Build history of the part. All positions in model axes, mm. Face numbers are marked on the shaded views. A direction names the side the tool comes from. Give positions to 0.01 mm unless a question says otherwise; leave off trailing zeros. Order: outer loops, then holes, each group sorted by start corner. A loop starts at its lowest first (then second) coordinate and runs counter-clockwise, first axis right, second up. Notation, with made-up numbers: (78, 67) - (111, 67) arc R23 ccw to (111, 100) - close; hole circle Ø3 at (88, -15.75). An arc over 180 degrees is marked (long way). Answer in a Markdown table with one row per item.
```python
from build123d import *

# Parameters (mm, degrees)
SKETCH1_W               = 50.8
SKETCH1_H               = 22.225
BOSS_EXTRUDE1_DEPTH     = 34.29
SKETCH2_R               = 18.034
CUT_EXTRUDE1_DEPTH      = 45.095938092
SKETCH3_W               = 20.32
SKETCH3_H               = 19.685
CUT_EXTRUDE2_DEPTH      = 63.289098213
SKETCH4_W               = 12.7
SKETCH4_H               = 19.05
CUT_EXTRUDE3_DEPTH      = 45.095938092
SKETCH7_W               = 68.58
SKETCH7_H               = 12.7
CUT_EXTRUDE5_DEPTH      = 49.113560718
CUT_EXTRUDE6_DEPTH      = 45.095938092
CUT_EXTRUDE6_DEPTH_BACK = 45.095938092
SKETCH9_W               = 5.08
SKETCH9_H               = 5.08
SKETCH6_W               = 33.625329213
SKETCH6_H               = 19.685
CUT_EXTRUDE4_DEPTH      = 45.095938092


with BuildPart() as part:
    # Sketch1 → Boss-Extrude1 (new, symmetric)
    with BuildSketch(Plane(origin=(0, 0, 0), x_dir=(0, 0, -1), z_dir=(1, 0, 0))):
        Rectangle(SKETCH1_W, SKETCH1_H)
    extrude(amount=BOSS_EXTRUDE1_DEPTH, both=True)

    # Sketch2 → Cut-Extrude1 (cut, through all)
    with BuildSketch(Plane(origin=(0, 0, 0), x_dir=(1, 0, 0), z_dir=(0, 0.819152044288991, 0.5735764363510473))):
        with Locations(Location((0, 0, 0), (0, 0, 233.158672775))):
            Circle(SKETCH2_R)
    extrude(amount=CUT_EXTRUDE1_DEPTH, mode=Mode.SUBTRACT)

    # Sketch3 → Cut-Extrude2 (cut, through all)
    with BuildSketch(Plane.XY.offset(25.4)):
        with Locations((0, 1.27)):
            Rectangle(SKETCH3_W, SKETCH3_H)
    extrude(amount=-CUT_EXTRUDE2_DEPTH, mode=Mode.SUBTRACT)

    # Sketch4 → Cut-Extrude3 (cut, through all)
    with BuildSketch(Plane(origin=(0, 0, 0), x_dir=(1, 0, 0), z_dir=(0, 1, 0))):
        Rectangle(SKETCH4_W, SKETCH4_H)
    extrude(amount=-CUT_EXTRUDE3_DEPTH, mode=Mode.SUBTRACT)

    # Sketch7 → Cut-Extrude5 (cut, through all)
    with BuildSketch(Plane(origin=(0, 11.1125, 0), x_dir=(1, 0, 0), z_dir=(0, 1, 0))):
        with Locations((0, 19.05)):
            Rectangle(SKETCH7_W, SKETCH7_H)
    extrude(amount=-CUT_EXTRUDE5_DEPTH, mode=Mode.SUBTRACT)

    # Sketch9 → Cut-Extrude6 (cut, two sides: drawn at the far end of the back side and taken through both)
    with BuildSketch(Plane.XY.offset(-CUT_EXTRUDE6_DEPTH_BACK)):
        with Locations((-31.75, -8.5725)):
            Rectangle(SKETCH9_W, SKETCH9_H)
        with Locations((31.75, -8.5725)):
            Rectangle(SKETCH9_W, SKETCH9_H)
    extrude(amount=CUT_EXTRUDE6_DEPTH + CUT_EXTRUDE6_DEPTH_BACK, mode=Mode.SUBTRACT)

    # Sketch6 → Cut-Extrude4 (cut, through all)
    with BuildSketch(Plane.XY):
        with Locations((-0.341373901, 1.27)):
            Rectangle(SKETCH6_W, SKETCH6_H)
    extrude(amount=CUT_EXTRUDE4_DEPTH, mode=Mode.SUBTRACT)


solid = part.part
```
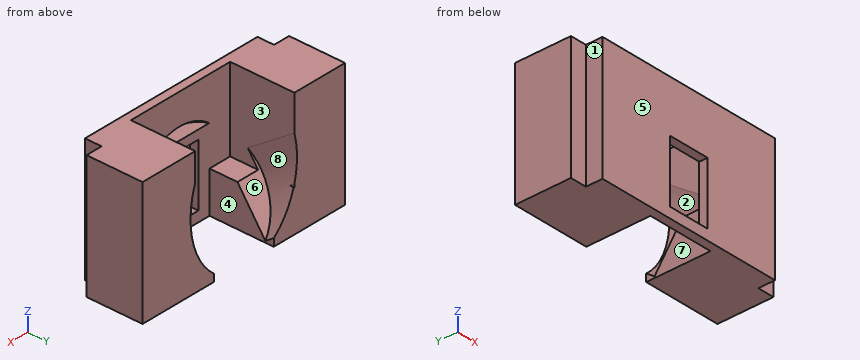
1. Probe line 1 (X direction, y = -5.75, z = 15); line 2 (X direction, y = 3, z = -5); line 3 (Y direction, x = -13, z = 18.5). List the from-to ranges inside material, lowest first.
Check result:
| item | result |
|---|---|
| line 1 | x = -34.29 to -17.15, 16.47 to 34.29 |
| line 2 | x = -34.29 to -10.16, 10.16 to 34.29 |
| line 3 | y = -11.11 to -8.57 |
2. Two-plate mould, pull along Y, no slides. Class the marked faces 5, 6, 7 and 8: +Y half, -Y half, draft (parallel to the pull), parting line (faces both ways), or undercut.
Check result:
| item | result |
|---|---|
| face 5 | -Y half |
| face 6 | undercut |
| face 7 | draft |
| face 8 | undercut |
3. Cut at B-B on x = -14.5. Write the cut outline in (y, z), and give its area (3 significant figures).
Check result:
| item | result |
|---|---|
| outline | (-11.11, -12.7) - (11.11, -12.7) - (11.11, -5.31) - (6.15, -8.78) - (0, 0) - (-8.57, 0) - (-8.57, 25.4) - (-11.11, 25.4) - close |
| area | 285 mm² |
4. Which spindle directions (+Z, -Z, +X, -X, +Y, -Y) get a long thin tool onto all of the face, cutting with end or side? Do the marked faces 1, 2, 3 and 4. Say none if no direction does.
Check result:
| item | result |
|---|---|
| face 1 | +Z, -Z, -X, -Y |
| face 2 | none |
| face 3 | +Z, +Y |
| face 4 | +Z, -Z, +Y |
5. Cut at A-A on x = 12.5. Write the cut outline in (y, z), and give its area (3 significant figures).
Check result:
| item | result |
|---|---|
| outline | (-11.11, -12.7) - (11.11, -12.7) - (11.11, -8.09) - (7.46, -10.65) - (0, 0) - (-8.57, 0) - (-8.57, 25.4) - (-11.11, 25.4) - close |
| area | 273 mm² |
6. Drop flat-ended pins along their axis: P1, Ø5.5, axis at x = 32.5, z = 14.5, coming from the -Y side; P2, Ø3, axis at y = -10, z = -3.5, coming from the +X side; P3, Ø2, axis at x = 7.5, y = -5.5, coming from the +Z side; P4, Ø1.9, axis at x = 14.5, y = -6.5, coming from the +Z side. Give the stop position or say it passes through.
Check result:
| item | result |
|---|---|
| P1 | stops at y = -6.03 |
| P2 | stops at x = 29.21 |
| P3 | passes through |
| P4 | stops at z = 0 |
